Autodesk Inventor part; units mm, degrees
ref_plane "YZ Plane" through (0, 0, 0) normal (1, 0, 0) x (0, 1, 0)
ref_plane "XZ Plane" through (0, 0, 0) normal (0, 1, 0) x (-1, 0, 0)
ref_plane "XY Plane" through (0, 0, 0) normal (0, 0, 1) x (1, 0, 0)
sketch "Sketch1" plane through (0, 0, 0) normal (0, 0, 1) x (1, 0, 0)
  circle A0 centre (0, 0) radius 8
  line L0 (0, 0) -> (16, 0) construction
  arc A1 (11.746, 0.9) -> (7.746, 2) centre (5.8068, -12.8741) ccw
  arc A2 (7.746, -2) -> (11.746, -0.9) centre (5.8068, 12.8741) ccw
  arc A3 (7.746, -2) -> (7.746, 2) centre (0, 0) ccw
  arc A4 (11.746, -0.9) -> (11.746, 0.9) centre (-8.2338, 0) ccw
  arc A5 (9.3948, 7.1075) -> (5.435, 5.8703) centre (11.8453, -7.691) ccw
  arc A6 (10.3679, 5.5932) -> (9.3948, 7.1075) centre (-6.9267, -4.4515) ccw
  arc A7 (7.5976, 2.5053) -> (10.3679, 5.5932) centre (-2.0753, 13.9698) ccw
  arc A8 (7.5976, 2.5053) -> (5.435, 5.8703) centre (0, 0) ccw
  arc A9 (4.0608, 11.0584) -> (1.3985, 7.8768) centre (14.123, -0.066) ccw
  arc A10 (5.6981, 10.3106) -> (4.0608, 11.0584) centre (-3.4204, -7.4897) ccw
  arc A11 (5.0371, 6.2151) -> (5.6981, 10.3106) centre (-9.2985, 10.6302) ccw
  arc A12 (5.0371, 6.2151) -> (1.3985, 7.8768) centre (0, 0) ccw
  arc A13 (-2.5625, 11.4983) -> (-3.082, 7.3825) centre (11.9167, 7.5799) ccw
  arc A14 (-0.7808, 11.7545) -> (-2.5625, 11.4983) centre (1.1718, -8.15) ccw
  arc A15 (0.8773, 7.9518) -> (-0.7808, 11.7545) centre (-13.5695, 3.9155) ccw
  arc A16 (0.8773, 7.9518) -> (-3.082, 7.3825) centre (0, 0) ccw
  arc A17 (-8.3721, 8.2876) -> (-6.584, 4.5443) centre (5.927, 12.8193) ccw
  arc A18 (-7.0118, 9.4664) -> (-8.3721, 8.2876) centre (5.392, -6.2227) ccw
  arc A19 (-3.561, 7.1637) -> (-7.0118, 9.4664) centre (-13.5323, -4.0423) ccw
  arc A20 (-3.561, 7.1637) -> (-6.584, 4.5443) centre (0, 0) ccw
  arc A21 (-11.5237, 2.4457) -> (-7.9957, 0.2633) centre (-1.9446, 13.9886) ccw
  arc A22 (-11.0166, 4.1728) -> (-11.5237, 2.4457) centre (7.9002, -2.3197) ccw
  arc A23 (-6.8687, 4.1013) -> (-11.0166, 4.1728) centre (-9.1987, -10.7167) ccw
  arc A24 (-6.8687, 4.1013) -> (-7.9957, 0.2633) centre (0, 0) ccw
  arc A25 (-11.0166, -4.1728) -> (-6.8687, -4.1013) centre (-9.1987, 10.7167) ccw
  arc A26 (-11.5237, -2.4457) -> (-11.0166, -4.1728) centre (7.9002, 2.3197) ccw
  arc A27 (-7.9957, -0.2633) -> (-11.5237, -2.4457) centre (-1.9446, -13.9886) ccw
  arc A28 (-7.9957, -0.2633) -> (-6.8687, -4.1013) centre (0, 0) ccw
  arc A29 (-7.0118, -9.4664) -> (-3.561, -7.1637) centre (-13.5323, 4.0423) ccw
  arc A30 (-8.3721, -8.2876) -> (-7.0118, -9.4664) centre (5.392, 6.2227) ccw
  arc A31 (-6.584, -4.5443) -> (-8.3721, -8.2876) centre (5.927, -12.8193) ccw
  arc A32 (-6.584, -4.5443) -> (-3.561, -7.1637) centre (0, 0) ccw
  arc A33 (-0.7808, -11.7545) -> (0.8773, -7.9518) centre (-13.5695, -3.9155) ccw
  arc A34 (-2.5625, -11.4983) -> (-0.7808, -11.7545) centre (1.1718, 8.15) ccw
  arc A35 (-3.082, -7.3825) -> (-2.5625, -11.4983) centre (11.9167, -7.5799) ccw
  arc A36 (-3.082, -7.3825) -> (0.8773, -7.9518) centre (0, 0) ccw
  arc A37 (5.6981, -10.3106) -> (5.0371, -6.2151) centre (-9.2985, -10.6302) ccw
  arc A38 (4.0608, -11.0584) -> (5.6981, -10.3106) centre (-3.4204, 7.4897) ccw
  arc A39 (1.3985, -7.8768) -> (4.0608, -11.0584) centre (14.123, 0.066) ccw
  arc A40 (1.3985, -7.8768) -> (5.0371, -6.2151) centre (0, 0) ccw
  arc A41 (10.3679, -5.5932) -> (7.5976, -2.5053) centre (-2.0753, -13.9698) ccw
  arc A42 (9.3948, -7.1075) -> (10.3679, -5.5932) centre (-6.9267, 4.4515) ccw
  arc A43 (5.435, -5.8703) -> (9.3948, -7.1075) centre (11.8453, 7.691) ccw
  arc A44 (5.435, -5.8703) -> (7.5976, -2.5053) centre (0, 0) ccw
  point P0 (11.7662, 0)
  point P1 (9.8984, 6.3613)
  point P2 (4.8879, 10.7029)
  point P3 (-1.6745, 11.6465)
  point P4 (-7.7052, 8.8923)
  point P5 (-11.2896, 3.3149)
  point P6 (-11.2896, -3.3149)
  point P7 (-7.7052, -8.8923)
  point P8 (-1.6745, -11.6465)
  point P9 (4.8879, -10.7029)
  point P10 (9.8984, -6.3613)
  dimension "d0" = 16
  dimension "d1" = 16
  dimension "d2" = 15
  dimension "d3" = 4
  dimension "d4" = 2
  dimension "d6" = 1.8
  dimension "d15" = 20
  dimension "d18" = 360
extrude "Extrusion1" add sketch "Sketch1" along normal blind 10
sketch "Sketch2" plane through (0, 0, 10) normal (0, 0, 1) x (1, 0, 0)
  circle A0 centre (0, 0) radius 3
  circle A1 centre (0, 0) radius 8
  dimension "d22" = 6
  dimension "d23" = 16
extrude "Extrusion2" add sketch "Sketch2" along normal blind 6
sketch "Sketch3" plane through (0, 0, 16) normal (0, 0, 1) x (1, 0, 0)
  circle A0 centre (0, 0) radius 3
extrude "Extrusion3" cut sketch "Sketch3" against normal through all
sketch "Sketch4" plane through (0, 0, 0) normal (1, 0, 0) x (0, 1, 0)
  circle A0 centre (0, 13) radius 1.5
  line L0 (8, 16) -> (-8, 16)
  point P0 (0, 0)
  dimension "d28" = 3
  dimension "d29" = 3
extrude "Extrusion4" cut sketch "Sketch4" along normal through all
properties part number "Motor Gear" material "ABS Plastic"
Here's how the part is built. I have some questions about the finished solid (model axes, mm). A direction names the side the tool comes from. Coordinates: 2 decimals unless noted, no trailing zeros. Order: outer loops, then holes, each group sorted by start corner. A loop starts at its lowest first (then second) coordinate and runs counter-clockwise, first axis right, second up. Notation, with made-up numbers: (25, -12) - (52, -12) arc R12 cw to (52, 2) - close; hole circle Ø1 at (-38, -34.75). An arc over 180 degrees is marked (long way). Use CSV: the item, a comma, the result in double quotes. Start each with the question number.
1. Suppose I cut it at D-D on z = 13.5. List the corners of the cut face in (x, y) for me, then the cut area to 3 significant figures.
2. I'm going to push flat-ended pins straight in: pin 1 (5 mm diameter, centred on y = 0, z = 13, fed in from +X); pin 2 (6 mm diameter, centred on y = 0.5, z = 4, fed in from -X); pin 3 (1.3 mm diameter, centred on x = 4.5, y = 8.5, fed in from +Z); pin 4 (6 mm diameter, centred on x = 8, z = 5.5, fed in from +Y). Where does each tip first touch, or does it pass through?
3. If we mould it in two halves opening along Z, with no side actions, what happens to faces 5 (the face through (5.26, -1.5, 12.93)), 6 (the face through (8, 5, 10)), 7 (the face through (-1.66, -11.65, 4.93))? For each: +Z half, -Z half, draft (parallel to the pull), parting line (faces both ways), or undercut.
4. Suppose I cut it at B-B on y = 6.75. List the corners of the cut face in (x, z) for me.
5. For faces 1 (the face through (-9.811, 1.217, 4.93)), 2 (the face through (-5.23, 8.45, 4.93)), 3 (the face through (9.81, -1.58, 4.93)), 4 (the face through (4, -9, 10)), which set-ups out of +Z, -Z, +X, -X, +Y, -Y let a thin tool reach every point of the face, with its end or its side?
6. Suppose I cut it at C-C on x = -10. List the corners of the cut face in (y, z) for me.
7. Please list where these lines run through material, in increasing order: line 1 (Y direction, x = -7, z = 4.75); line 2 (Z direction, x = 4.05, y = 0); line 3 (Y direction, x = 0, z = 8.5). Write a range as from..to.
8. Suppose I cut it at A-A on x = 0. List the corners of the cut face in (y, z) for me.
Output:
1,outline,"(2.65, -1.41) arc R3 cw (long way) to (2.65, 1.41) - (7.87, 1.41) arc R8 ccw (long way) to (7.87, -1.41) - close"
1,area,"158 mm2"
2,pin 1,"stops at x = 8"
2,pin 2,"stops at x = -11.52"
2,pin 3,"stops at z = 10"
2,pin 4,"stops at y = 10.65"
3,face 5,"undercut"
3,face 6,"+Z half"
3,face 7,"draft"
4,outline,"(-7.79, 0) - (5.19, 0) - (5.19, 10) - (4.29, 10) - (4.29, 16) - (-4.29, 16) - (-4.29, 10) - (-7.79, 10) - close; (7.79, 0) - (9.64, 0) - (9.64, 10) - (7.79, 10) - close"
5,face 1,"+Z, -Z, -X"
5,face 2,"+Z, -Z, +Y"
5,face 3,"+Z, -Z, +X"
5,face 4,"+Z, +X, -Y"
6,outline,"(-4.26, 0) - (-1.34, 0) - (-1.34, 10) - (-4.26, 10) - close; (1.34, 0) - (4.26, 0) - (4.26, 10) - (1.34, 10) - close"
7,line 1,"y = -9.46..-5.21, -4.12..4.12, 5.21..9.46"
7,line 2,"z = 0..11.5, 14.5..16"
7,line 3,"y = -10.31..-3, 3..10.31"
8,outline,"(-10.31, 0) - (-3, 0) - (-3, 16) - (-8, 16) - (-8, 10) - (-10.31, 10) - close; (3, 0) - (10.31, 0) - (10.31, 10) - (8, 10) - (8, 16) - (3, 16) - close"
